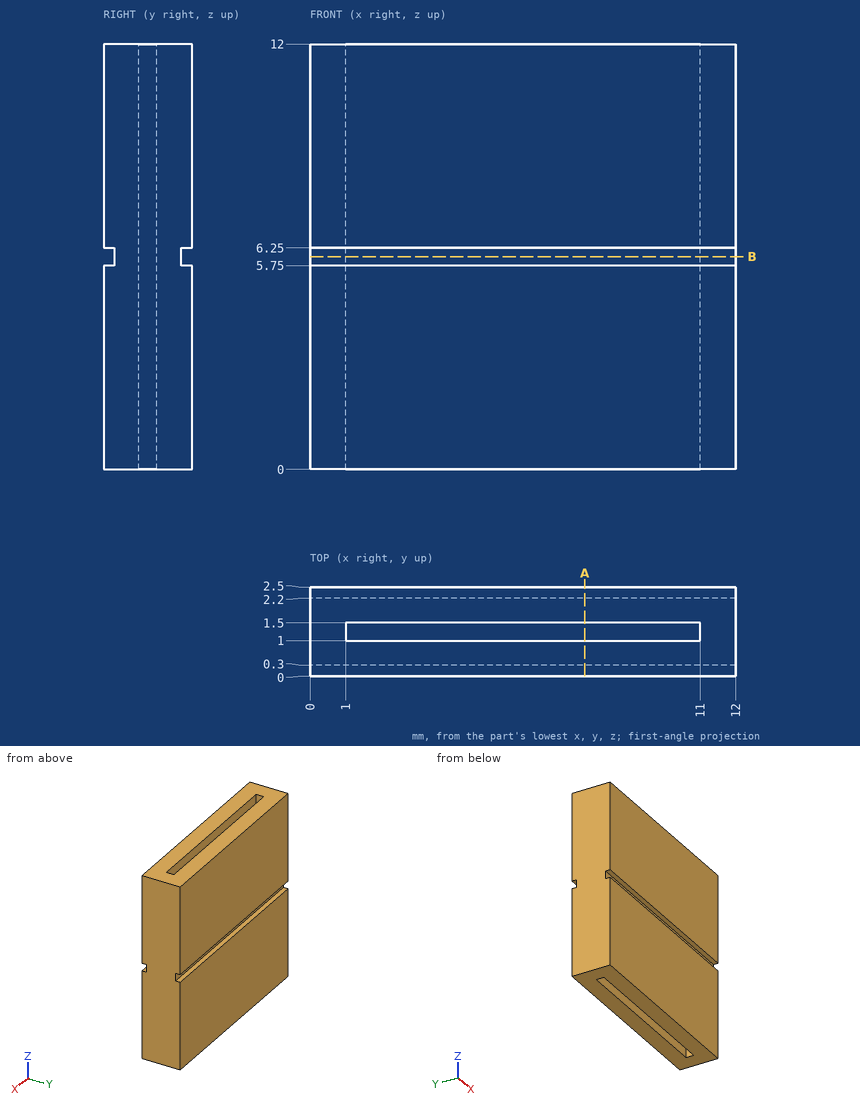
For this review, use the dimensioned drawing (mm, ordinates from the lowest corner) and the shaded views. Round coordinates to 2 decimals unless told otherwise and drop trailing zeros. Order: outer loops, then holes, each group sorted by start corner. A loop starts at its lowest first (then second) coordinate and runs counter-clockwise, first axis right, second up. Notation, with made-up numbers: (10.5, 30) -> (65.5, 30) arc R14 cw to (65.5, 47) -> close; hole circle Ø7 at (68, -16). An arc over 180 degrees is marked (long way). Put each result on its own line as item: value.
Q1. Add section A-A on x = 7.75. Write out the cut boundary in (y, z), plus the area to 3 significant figures.
Check result:
outline: (0, 0) -> (1, 0) -> (1, 12) -> (0, 12) -> (0, 6.25) -> (0.3, 6.25) -> (0.3, 5.75) -> (0, 5.75) -> close; (1.5, 0) -> (2.5, 0) -> (2.5, 5.75) -> (2.2, 5.75) -> (2.2, 6.25) -> (2.5, 6.25) -> (2.5, 12) -> (1.5, 12) -> close
area: 23.7 mm2
Q2. Add section B-B on z = 6. Write out the cut boundary in (x, y), plus the area to 3 significant figures.
Check result:
outline: (0, 0.3) -> (12, 0.3) -> (12, 2.2) -> (0, 2.2) -> close; hole (1, 1) -> (11, 1) -> (11, 1.5) -> (1, 1.5) -> close
area: 17.8 mm2
Q3. For probe 1 along Y at (x, z) = (5, 4.5); probe 2 along X at (y, z) = (1.1, 3.25), list the stretches that pass through material, from the lowest coordinate up. Write a range as [from, to].
Check result:
probe 1: [0, 1], [1.5, 2.5]
probe 2: [0, 1], [11, 12]
